The model under review builds one solid part; all positions refer to its coordinate system, in mm. Round coordinates to 2 decimals unless told otherwise and drop trailing zeros. Order: outer loops, then holes, each group sorted by start corner. A loop starts at its lowest first (then second) coordinate and runs counter-clockwise, first axis right, second up. Notation, with made-up numbers: M 38.25,85.5 L 56.25,85.5 A28 cw 56.25,114.5 Z; hole C 68,27 d5. An arc over 180 degrees is marked long. Answer as a JSON object with one key per item and string values. Group by question number.
1. Add section B-B on y = 66. State the section outline as (x, z) points, and give its area (3 significant figures).
2. Add section C-C on z = 4.55. Give the number of separate pieces and of enclosed holes in the cut face, and give its area (3 significant figures).
3. Add section D-D on x = 32. State the section outline as (y, z) points, and give its area (3 significant figures).
4. Add section A-A on x = -49.5. State the section outline as (y, z) points.
5. Clearance check with flat-ended pins moving along their axes: P1, Ø10, axis at x = 42.5, y = -19.5, coming from the -Z side; P2, Ø5, axis at x = 40.4, y = -25.77, coming from the +Z side; P3, Ø1.8, axis at x = -52.5, z = 3, coming from the +Y side; P4, Ø3, axis at x = 43, z = 4.5, coming from the +Y side. State where each tip first meets the part, or that it passes through.
6. To check wall thickness, follow probe 1 along X at (y, z) = (-26, 1.15); probe 2 along Y at (x, z) = (7.5, 4.65); probe 3 along X at (y, z) = (21.5, 1.2). State the ranges of each line that lie inside material, in increasing order. Write a range as [from, to].
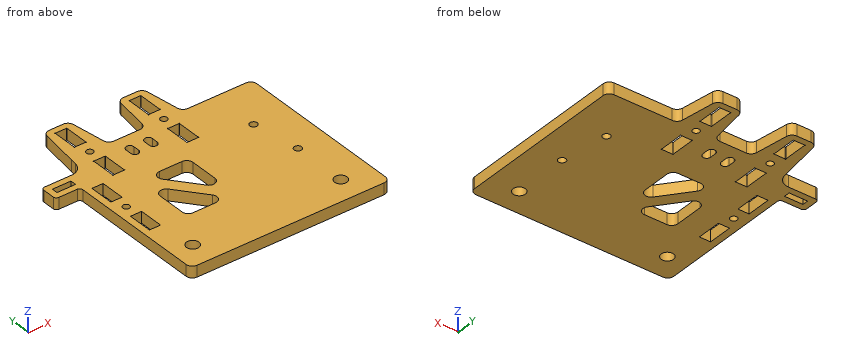
```python
from build123d import *

# Parameters (mm, degrees)
SKETCH1_R           = 3.175
SKETCH1_R_2         = 1.7526
SKETCH1_W           = 5.742
SKETCH1_H           = 12.5
BOSS_EXTRUDE1_DEPTH = 5.842
CUT_EXTRUDE2_DEPTH  = 77.987395934
BOSS_EXTRUDE2_DEPTH = 5.842
FILLET1_R           = 3.175
SKETCH5_R           = 1.7526
CUT_EXTRUDE3_DEPTH  = 94.593735754
CUT_EXTRUDE4_DEPTH  = 94.593735754
FILLET2_R           = 3.175
CUT_EXTRUDE8_DEPTH  = 94.593735754
FILLET3_R           = 3.175
SKETCH11_R          = 1.9199987
CUT_EXTRUDE9_DEPTH  = 94.593735754
CUT_EXTRUDE10_DEPTH = 94.593735754
BOSS_EXTRUDE3_START = -5.842
SKETCH14_W          = 9.525
SKETCH14_H          = 3.048
BOSS_EXTRUDE3_DEPTH = 5.842
FILLET4_R           = 1.5875
FILLET5_R           = 6.35


with BuildPart() as part:
    # Sketch1 → Boss-Extrude1 (new body)
    with BuildSketch(Plane.XY):
        Polygon((51.85043079, -38.469674457), (-46.57456921, -38.469674457), (-46.57456921, 34.555325543), (-46.57456921, 52.615919343), (51.85043079, 52.615919343), (55.89718419, 52.615919343), (55.89718419, -38.469674457), align=None)
        with Locations((-35.79681581, -25.769674457)):
            Circle(SKETCH1_R, mode=Mode.SUBTRACT)
        with Locations((40.40318419, -25.769674457)):
            Circle(SKETCH1_R, mode=Mode.SUBTRACT)
        with Locations((-40.22456921, 12.330325543)):
            Circle(SKETCH1_R_2, mode=Mode.SUBTRACT)
        with Locations((-40.22456921, -0.369674457)):
            Rectangle(SKETCH1_W, SKETCH1_H, mode=Mode.SUBTRACT)
        with Locations((-40.22456921, 25.030325543)):
            Rectangle(SKETCH1_W, SKETCH1_H, mode=Mode.SUBTRACT)
    extrude(amount=BOSS_EXTRUDE1_DEPTH)

    # Sketch3 → Cut-Extrude2 (cut, through all)
    with BuildSketch(Plane.XY.offset(5.842)):
        with BuildLine():
            Line((-24.73850671, 33.565919343), (-30.31063171, 33.565919343))
            ThreePointArc((-30.31063171, 33.565919343), (-30.649385711, 33.425602841), (-30.50906921, 33.764356843))
            Line((-30.50906921, 33.764356843), (-30.50906921, 46.067481843))
            ThreePointArc((-30.50906921, 46.067481843), (-30.649385711, 46.406235845), (-30.31063171, 46.265919343))
            Line((-30.31063171, 46.265919343), (-24.73850671, 46.265919343))
            ThreePointArc((-24.73850671, 46.265919343), (-24.399752708, 46.406235845), (-24.54006921, 46.067481843))
            Line((-24.54006921, 46.067481843), (-24.54006921, 33.764356843))
            ThreePointArc((-24.54006921, 33.764356843), (-24.399752708, 33.425602841), (-24.73850671, 33.565919343))
        make_face()
        with BuildLine():
            Line((13.55993079, 33.764356843), (13.55993079, 46.067481843))
            ThreePointArc((13.55993079, 46.067481843), (13.700247292, 46.406235845), (13.36149329, 46.265919343))
            Line((13.36149329, 46.265919343), (7.78936829, 46.265919343))
            ThreePointArc((7.78936829, 46.265919343), (7.450614289, 46.406235845), (7.59093079, 46.067481843))
            Line((7.59093079, 46.067481843), (7.59093079, 33.764356843))
            ThreePointArc((7.59093079, 33.764356843), (7.450614289, 33.425602841), (7.78936829, 33.565919343))
            Line((7.78936829, 33.565919343), (13.36149329, 33.565919343))
            ThreePointArc((13.36149329, 33.565919343), (13.700247292, 33.425602841), (13.55993079, 33.764356843))
        make_face()
    extrude(amount=-CUT_EXTRUDE2_DEPTH, mode=Mode.SUBTRACT)

    # Sketch4 → Boss-Extrude2 (add)
    # profile 1 of 2: a face of its own
    with BuildSketch(Plane.XY.offset(5.842)):
        Polygon((1.036619808, 52.615919343), (4.22543079, 74.840919343), (16.92543079, 74.840919343), (20.086619808, 52.615919343), align=None)
        with BuildLine():
            Line((13.36149329, 71.665919343), (7.78936829, 71.665919343))
            ThreePointArc((7.78936829, 71.665919343), (7.450614289, 71.806235845), (7.59093079, 71.467481843))
            Line((7.59093079, 71.467481843), (7.59093079, 59.164356843))
            ThreePointArc((7.59093079, 59.164356843), (7.450614289, 58.825602841), (7.78936829, 58.965919343))
            Line((7.78936829, 58.965919343), (13.36149329, 58.965919343))
            ThreePointArc((13.36149329, 58.965919343), (13.700247292, 58.825602841), (13.55993079, 59.164356843))
            Line((13.55993079, 59.164356843), (13.55993079, 71.467481843))
            ThreePointArc((13.55993079, 71.467481843), (13.700247292, 71.806235845), (13.36149329, 71.665919343))
        make_face(mode=Mode.SUBTRACT)
    # profile 2 of 2: a face of its own
    with BuildSketch(Plane.XY.offset(5.842)):
        Polygon((-37.035758227, 52.615919343), (-17.985758227, 52.615919343), (-21.17456921, 74.840919343), (-33.87456921, 74.840919343), align=None)
        with BuildLine():
            Line((-24.54006921, 71.467481843), (-24.54006921, 59.164356843))
            ThreePointArc((-24.54006921, 59.164356843), (-24.399752708, 58.825602841), (-24.73850671, 58.965919343))
            Line((-24.73850671, 58.965919343), (-30.31063171, 58.965919343))
            ThreePointArc((-30.31063171, 58.965919343), (-30.649385711, 58.825602841), (-30.50906921, 59.164356843))
            Line((-30.50906921, 59.164356843), (-30.50906921, 71.467481843))
            ThreePointArc((-30.50906921, 71.467481843), (-30.649385711, 71.806235845), (-30.31063171, 71.665919343))
            Line((-30.31063171, 71.665919343), (-24.73850671, 71.665919343))
            ThreePointArc((-24.73850671, 71.665919343), (-24.399752708, 71.806235845), (-24.54006921, 71.467481843))
        make_face(mode=Mode.SUBTRACT)
    extrude(amount=-BOSS_EXTRUDE2_DEPTH)

    # Fillet1
    fillet1_edges = [part.edges().sort_by_distance(p)[0] for p in [
        (20.086619808, 52.615919343, 2.921),
        (16.92543079, 74.840919343, 2.921),
        (4.22543079, 74.840919343, 2.921),
        (1.036619808, 52.615919343, 2.921),
        (-17.985758227, 52.615919343, 2.921),
        (-21.17456921, 74.840919343, 2.921),
        (-33.87456921, 74.840919343, 2.921),
    ]]
    fillet(fillet1_edges, radius=FILLET1_R)

    # Sketch5 → Cut-Extrude3 (cut, through all)
    with BuildSketch(Plane.XY.offset(5.842)):
        with Locations((-27.52456921, 52.615919343)):
            Circle(SKETCH5_R)
        with Locations((10.57543079, 52.615919343)):
            Circle(SKETCH5_R)
    extrude(amount=-CUT_EXTRUDE3_DEPTH, mode=Mode.SUBTRACT)

    # Sketch6 → Cut-Extrude4 (cut, through all)
    with BuildSketch(Plane.XY.offset(5.842)):
        Polygon((-37.035758227, 52.615919343), (-39.167245046, 37.630325543), (-46.57456921, 37.630325543), (-46.57456921, 52.615919343), align=None)
    extrude(amount=-CUT_EXTRUDE4_DEPTH, mode=Mode.SUBTRACT)

    # Fillet2
    fillet2_edges = [part.edges().sort_by_distance(p)[0] for p in [
        (-39.167245046, 37.630325543, 2.921),
        (-46.57456921, 37.630325543, 2.921),
        (-46.57456921, -38.469674457, 2.921),
        (55.89718419, 52.615919343, 2.921),
        (55.89718419, -38.469674457, 2.921),
    ]]
    fillet(fillet2_edges, radius=FILLET2_R)

    # Sketch10 → Cut-Extrude8 (cut, through all)
    with BuildSketch(Plane.XY.offset(5.842)):
        Polygon((-20.587585319, 24.040919343), (0.74643079, 24.040919343), (0.74643079, -2.626600794), align=None)
        Polygon((-24.65356921, 18.958439479), (-24.65356921, -7.709080657), (-3.3195531, -7.709080657), align=None)
    extrude(amount=-CUT_EXTRUDE8_DEPTH, mode=Mode.SUBTRACT)

    # Fillet3
    fillet3_edges = [part.edges().sort_by_distance(p)[0] for p in [
        (0.74643079, 24.040919343, 2.921),
        (0.74643079, -2.626600794, 2.921),
        (-20.587585319, 24.040919343, 2.921),
        (-3.3195531, -7.709080657, 2.921),
        (-24.65356921, -7.709080657, 2.921),
        (-24.65356921, 18.958439479, 2.921),
    ]]
    fillet(fillet3_edges, radius=FILLET3_R)

    # Sketch11 → Cut-Extrude9 (cut, through all)
    with BuildSketch(Plane.XY.offset(5.842)):
        with Locations((36.84718419, 27.215919343)):
            Circle(SKETCH11_R)
        with Locations((40.44717699, 2.565930543)):
            Circle(SKETCH11_R)
    extrude(amount=-CUT_EXTRUDE9_DEPTH, mode=Mode.SUBTRACT)

    # Sketch12 → Cut-Extrude10 (cut, through all)
    with BuildSketch(Plane.XY.offset(5.842)):
        with BuildLine():
            Line((-5.71206921, 41.291183898), (-5.71206921, 44.466183898))
            ThreePointArc((-5.71206921, 44.466183898), (-3.71206921, 46.466183898), (-1.71206921, 44.466183898))
            Line((-1.71206921, 44.466183898), (-1.71206921, 41.291183898))
            ThreePointArc((-1.71206921, 41.291183898), (-3.71206921, 39.291183898), (-5.71206921, 41.291183898))
        make_face()
        with BuildLine():
            Line((-11.23706921, 41.291183898), (-11.23706921, 44.466183898))
            ThreePointArc((-11.23706921, 44.466183898), (-13.23706921, 46.466183898), (-15.23706921, 44.466183898))
            Line((-15.23706921, 44.466183898), (-15.23706921, 41.291183898))
            ThreePointArc((-15.23706921, 41.291183898), (-13.23706921, 39.291183898), (-11.23706921, 41.291183898))
        make_face()
    extrude(amount=-CUT_EXTRUDE10_DEPTH, mode=Mode.SUBTRACT)

    # Sketch14 → Boss-Extrude3 (add)
    with BuildSketch(Plane.XY.offset(5.842).offset(BOSS_EXTRUDE3_START)):
        with BuildLine():
            Line((-42.661085862, 37.630325543), (-42.661085862, 34.455325543))
            Line((-42.661085862, 34.455325543), (-59.27456921, 34.455325543))
            Line((-59.27456921, 34.455325543), (-59.27456921, 37.630325543))
            Line((-59.27456921, 37.630325543), (-59.27456921, 43.853325543))
            Line((-59.27456921, 43.853325543), (-38.282112121, 43.853325543))
            Line((-38.282112121, 43.853325543), (-38.779239988, 40.358227091))
            ThreePointArc((-38.779239988, 40.358227091), (-39.84160667, 38.40739283), (-41.922602515, 37.630325543))
            Line((-41.922602515, 37.630325543), (-42.661085862, 37.630325543))
        make_face()
        with Locations((-51.33706921, 39.154325543)):
            Rectangle(SKETCH14_W, SKETCH14_H, mode=Mode.SUBTRACT)
    extrude(amount=BOSS_EXTRUDE3_DEPTH)

    # Fillet4
    fillet4_edges = [part.edges().sort_by_distance(p)[0] for p in [
        (-46.57456921, 34.455325543, 2.921),
        (-59.27456921, 43.853325543, 2.921),
        (-59.27456921, 34.455325543, 2.921),
    ]]
    fillet(fillet4_edges, radius=FILLET4_R)

    # Fillet5
    fillet5_edges = [part.edges().sort_by_distance(p)[0] for p in [
        (-38.282112121, 43.853325543, 2.921),
    ]]
    fillet(fillet5_edges, radius=FILLET5_R)


solid = part.part
```
Recorded:
{
 "1": {"outline": "M -35.13,0 L -30.51,0 L -30.51,5.84 L -35.13,5.84 Z; M -24.54,0 L -19.91,0 L -19.91,5.84 L -24.54,5.84 Z; M 2.96,0 L 7.59,0 L 7.59,5.84 L 2.96,5.84 Z; M 13.56,0 L 18.18,0 L 18.18,5.84 L 13.56,5.84 Z", "area": "108 mm²"},
 "2": {"separate pieces": "1", "enclosed holes": "18", "area": "8,920 mm²"},
 "3": {"outline": "M -38.47,0 L 52.62,0 L 52.62,5.84 L -38.47,5.84 Z", "area": "532 mm²"},
 "4": {"outline": "M 34.46,0 L 37.63,0 L 37.63,5.84 L 34.46,5.84 Z; M 40.68,0 L 43.85,0 L 43.85,5.84 L 40.68,5.84 Z"},
 "5": {"P1": "stops at z = 0", "P2": "passes through", "P3": "stops at y = 43.85", "P4": "stops at y = 52.62"},
 "6": {"probe 1": "x = [-46.57, -38.96], [-32.63, 37.24], [43.57, 55.9]", "probe 2": "y = [-38.47, 33.39], [33.74, 46.09], [46.44, 58.79], [59.14, 71.49], [71.84, 74.84]", "probe 3": "x = [-46.57, -43.1], [-37.35, -17.09], [0.68, 55.9]"}
}
